Can you work these out from the model? Positions are in its coordinate system, mm. A direction names the side the tool comes from. Round coordinates to 2 decimals unless told otherwise and drop trailing zeros. Order: outer loops, then holes, each group sorted by start corner. A loop starts at its lowest first (then second) coordinate and runs counter-clockwise, first axis right, second up. Notation, with made-up numbers: (16, 89) - (23, 89) arc R35 cw to (23, 126) - close; hole circle Ø10 at (61.25, 62.25). An arc over 180 degrees is marked (long way). Write item = value, one per line.
Autodesk Inventor part; units mm, degrees
ref_plane "YZ Plane" through (0, 0, 0) normal (1, 0, 0) x (0, 1, 0)
ref_plane "XZ Plane" through (0, 0, 0) normal (0, 1, 0) x (-1, 0, 0)
ref_plane "XY Plane" through (0, 0, 0) normal (0, 0, 1) x (1, 0, 0)
sketch "Esboço1" plane through (0, 0, 0) normal (0, 0, 1) x (1, 0, 0)
  line L0 (-162.5, -7.5) -> (-117.5, -7.5) construction
  line L1 (162.5, -7.5) -> (162.5, 7.5)
  line L2 (162.5, 7.5) -> (-117.5, 7.5)
  line L3 (-162.5, 7.5) -> (-162.5, 5) construction
  line L4 (-162.5, -7.5) -> (162.5, 7.5) construction
  line L5 (162.5, -7.5) -> (-162.5, 7.5) construction
  line L6 (-162.5, -5) -> (-117.5, -5)
  line L7 (-117.5, 5) -> (-162.5, 5)
  line L8 (-117.5, 5) -> (-117.5, 7.5)
  line L9 (-117.5, -5) -> (-117.5, -7.5)
  line L10 (-117.5, 5) -> (-117.5, -5) construction
  line L11 (-117.5, 0) -> (0, 0) construction
  line L12 (-162.5, 5) -> (-162.5, -5)
  line L13 (-162.5, -5) -> (-162.5, -7.5) construction
  line L14 (-117.5, -7.5) -> (162.5, -7.5)
  line L15 (-117.5, 7.5) -> (-162.5, 7.5) construction
  dimension "d0" = 325
  dimension "d1" = 15
  dimension "d2" = 10
  dimension "d3" = 45
extrude "Extrusão1" add sketch "Esboço1" along normal mid plane 50
sketch "Esboço2" plane through (-162.5, 5, 25) normal (0, 1, 0) x (1, 0, 0)
  line L0 (0, 0) -> (0, 50)
  line L1 (45, 50) -> (45, 0)
  circle A0 centre (22.5, 35) radius 5
  circle A1 centre (22.5, 15) radius 5
  line L2 (22.5, 15) -> (22.5, 35)
  line L3 (0, 50) -> (45, 50)
  line L4 (22.5, 50) -> (22.5, 74.6859)
  line L5 (22.5, 25) -> (-20.9828, 25) construction
  line L6 (0, 25) -> (-37.1648, 25) construction
  point P0 (162.5, 25)
  dimension "d14" = 10
  dimension "d15" = 10
  dimension "d16" = 20
extrude "Extrusão2" cut sketch "Esboço2" against normal up to surface (10 mm away)
sketch "ref. Motor" plane through (-117.5, -7.5, 25) normal (0, -1, 0) x (1, 0, 0)
  line L0 (280, -50) -> (280, 0)
  line L1 (280, -25) -> (270, -25) construction
  line L2 (270, -25) -> (270, 54.6764) construction
  point P0 (117.5, -25)
  dimension "d13" = 10
equation "\"d15\" = d14"
properties part number "Pás - Hastes"
(1) If we section it at A-A (z = -10): Write out the boundary of the cut face in (x, y).
Computed:
outline = (-162.5, -5) - (-145, -5) - (-145, 5) - (-162.5, 5) - close; (-135, -5) - (-117.5, -5) - (-117.5, -7.5) - (162.5, -7.5) - (162.5, 7.5) - (-117.5, 7.5) - (-117.5, 5) - (-135, 5) - close
(2) On a 3-axis mill with a long thin cutter (end or side, diameter ignored), from which of +Z, -Z, +X, -X, +Y, -Y can I reach the whole of each face in a straight line? I mean faces 5 (the face through (-140, -5, 0)), 6 (the face through (-162.5, 0, 0)). Say none if no direction works.
Computed:
face_5 = +Z, -Z, -X, -Y
face_6 = +Z, -Z, -X, +Y, -Y
(3) If we section it at C-C (z = 19.5): Write out the boundary of the cut face in (x, y), plus the area to 3 significant figures.
Computed:
outline = (-162.5, -5) - (-117.5, -5) - (-117.5, -7.5) - (162.5, -7.5) - (162.5, 7.5) - (-117.5, 7.5) - (-117.5, 5) - (-162.5, 5) - close
area = 4,650 mm^2
(4) If I drill on line 1 (Z direction, x = -140, y = -2); line 2 (X direction, y = -2.5, z = 10); line 3 (Y direction, x = -118.5, z = -10.5), over which ranges is the centre line in solid material (lowest first)? Write a range as from..to.
Computed:
line_1 = -25..-15, -5..5, 15..25
line_2 = -162.5..-145, -135..162.5
line_3 = -5..5
(5) Thinking about a two-plate mould opening in X: for faces 1 (the face through (-145, 0, -10)), 2 (the face through (-140, 5, 0)), 3 (the face through (-144, 0, 13)), 4 (the face through (162.5, 0, 0)), which applies, +X half, -X half, draft (parallel to the pull), parting line (faces both ways), or undercut?
Computed:
face_1 = undercut
face_2 = draft
face_3 = undercut
face_4 = +X half
(6) Will these pins go through, and if not, where does the flat tip stop? P1, Ø16, axis at x = -140, z = 10, coming from the -Y side; P2, Ø2, axis at y = 6.5, z = -10.5, coming from the -X side.
Computed:
P1 = -5
P2 = -117.5
(7) If we section it at B-B (x = -140): Write out the boundary of the cut face in (y, z), plus the area to 3 significant figures.
Computed:
outline = (-5, -25) - (5, -25) - (5, -15) - (-5, -15) - close; (-5, -5) - (5, -5) - (5, 5) - (-5, 5) - close; (-5, 15) - (5, 15) - (5, 25) - (-5, 25) - close
area = 300 mm^2
